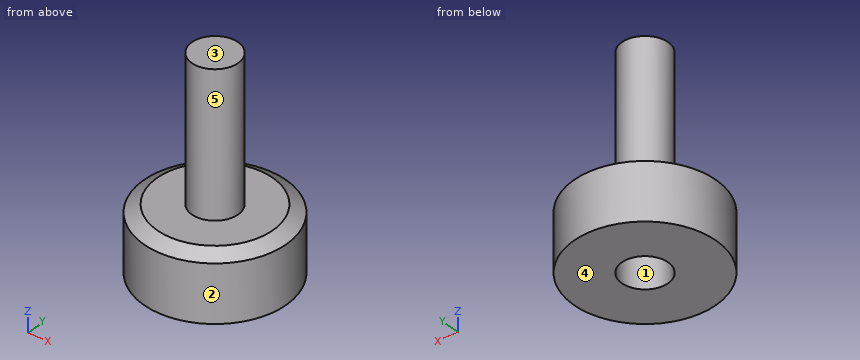
from build123d import *

# Parameters (mm, degrees)
F0_W   = 3.25
F0_H   = 20
F0_H_2 = 3
F0_H_3 = 1.0746234533


with BuildPart() as f1:
    # F0 (on Front) → F1 (revolve)
    with BuildSketch(Plane.XZ):
        with Locations((-22.1763077103, 19.0746234533)):
            Rectangle(F0_W, F0_H)
        Polygon((-23.8013077103, 8), (-30.5513077103, 8), (-30.5513077103, 0), (-23.8013077103, 0), (-23.8013077103, 5), align=None)
        Polygon((-28.6900052902, 9.0746234533), (-30.5513077103, 8), (-23.8013077103, 8), (-23.8013077103, 9.0746234533), align=None)
        with Locations((-22.1763077103, 6.5)):
            Rectangle(F0_W, F0_H_2)
        with Locations((-22.1763077103, 8.5373117267)):
            Rectangle(F0_W, F0_H_3)
    revolve(axis=Axis((-20.5513077103, 0, 19.0746234533), (0, 0, 1)))


solid = f1.part
Design review of the part built by this model. Coordinates are the model's own, in mm. Face numbers are marked on the shaded views. A direction names the side the tool comes from. Round coordinates to 2 decimals unless told otherwise and drop trailing zeros. Write each loop counter-clockwise with the first axis right and the second up, starting at its lowest first coordinate (ties: lowest second). Pieces come first, ordered by that corner, then holes.
Item 1: Consider section A-A on y = 0. Give the boundary of the cut face in (x, z).
Item 2: Wall thickness on L1, parallel to X at y = 0, z = 3.4; L2, parallel to Z at x = -14.5, y = 1.5; L3, parallel to Z at x = -20.25, y = 1: over which ranges is each line inside the solid? List them lowest first.
Item 3: Consider section B-B on z = 27.25. Give the boundary of the cut face in (x, y), and give its area (3 significant figures).
Item 4: Consider section C-C on z = 4. Give the boundary of the cut face in (x, y), and give its area (3 significant figures).
Item 5: For the marked faces 4 and 5, list the 3-axis set-ups (+Z, -Z, +X, -X, +Y, -Y) from which the entire face can be reached by the end or side of a thin tool; tool diameter is ignored.
Item 6: For pin 1 Ø6 at (y, z) = (7.5, 6.5) entering from -X; pin 2 Ø10 at (x, z) = (-23.5, 21) entering from -Y; pin 3 Ø3 at (x, z) = (-24, 5) entering from -Y, all flat-tipped, find the tip position at first contact; note any pin that passes through.
Item 7: Draft analysis for pull direction Y (two halves, no side actions). For the marked faces 1, 2 and 3, state which applies: released by +Y, released by -Y, zero draft, split by the parting line, or undercut.
Check values:
1. outline: (-30.55, 0) - (-23.8, 0) - (-23.8, 5) - (-17.3, 5) - (-17.3, 0) - (-10.55, 0) - (-10.55, 8) - (-12.41, 9.07) - (-17.3, 9.07) - (-17.3, 29.07) - (-23.8, 29.07) - (-23.8, 9.07) - (-28.69, 9.07) - (-30.55, 8) - close
2. L1: x = -30.55 to -23.8, -17.3 to -10.55
2. L2: z = 0 to 9.07
2. L3: z = 5 to 29.07
3. outline: circle Ø6.5 at (-20.55, 0)
3. area: 33.2 mm2
4. outline: circle Ø20 at (-20.55, 0); hole circle Ø6.5 at (-20.55, 0)
4. area: 281 mm2
5. face 4: -Z, +X, -X, +Y, -Y
5. face 5: +Z
6. pin 1: stops at x = -29.48
6. pin 2: stops at y = -3.25
6. pin 3: stops at y = -9.81
7. face 1: undercut
7. face 2: split by the parting line
7. face 3: zero draft
